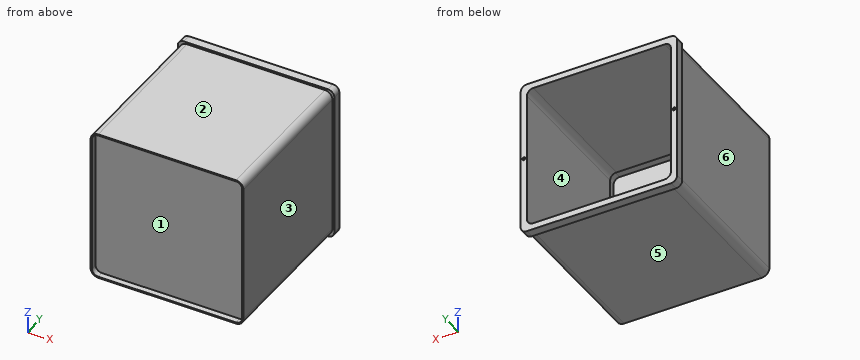
from build123d import *

# Parameters (mm, degrees)
EXTRUDE_1_DEPTH   = 125
EXTRUDE_1_2_DEPTH = 1
EXTRUDE_2_DEPTH   = 115
SKETCH_5_R        = 1.25
EXTRUDE_3_DEPTH   = 1
EXTRUDE_4_REACH   = 155.093
EXTRUDE_START     = -1
EXTRUDE_5_DEPTH   = 1


with BuildPart() as part:
    # Sketch 1 → Extrude 1 (new body)
    with BuildSketch(Plane(origin=(0, 0, 0), x_dir=(1, 0, 0), z_dir=(0, 1, 0))):
        with BuildLine():
            Line((55, -61), (-55, -61))
            ThreePointArc((-55, -61), (-59.242640687, -59.242640687), (-61, -55))
            Line((-61, -55), (-61, 55))
            ThreePointArc((-61, 55), (-59.242640687, 59.242640687), (-55, 61))
            Line((-55, 61), (55, 61))
            ThreePointArc((55, 61), (59.242640687, 59.242640687), (61, 55))
            Line((61, 55), (61, -55))
            ThreePointArc((61, -55), (59.242640687, -59.242640687), (55, -61))
        make_face()
        with BuildLine():
            Line((55, -60), (-55, -60))
            ThreePointArc((-55, -60), (-58.535533906, -58.535533906), (-60, -55))
            Line((-60, -55), (-60, 55))
            ThreePointArc((-60, 55), (-58.535533906, 58.535533906), (-55, 60))
            Line((-55, 60), (55, 60))
            ThreePointArc((55, 60), (58.535533906, 58.535533906), (60, 55))
            Line((60, 55), (60, -55))
            ThreePointArc((60, -55), (58.535533906, -58.535533906), (55, -60))
        make_face(mode=Mode.SUBTRACT)
    extrude(amount=EXTRUDE_1_DEPTH)

    # Sketch 2 → Extrude 1 2 (add)
    with BuildSketch(Plane(origin=(0, 5, 0), x_dir=(1, 0, 0), z_dir=(0, 1, 0))):
        with BuildLine():
            Line((-60, 55), (-60, -55))
            ThreePointArc((-60, -55), (-58.535533906, -58.535533906), (-55, -60))
            Line((-55, -60), (55, -60))
            ThreePointArc((55, -60), (58.535533906, -58.535533906), (60, -55))
            Line((60, -55), (60, 55))
            ThreePointArc((60, 55), (58.535533906, 58.535533906), (55, 60))
            Line((55, 60), (-55, 60))
            ThreePointArc((-55, 60), (-58.535533906, 58.535533906), (-60, 55))
        make_face()
    extrude(amount=EXTRUDE_1_2_DEPTH)



with BuildPart() as body_2:
    # Sketch 4 → Extrude 2 (new body)
    with BuildSketch(Plane(origin=(0, 15, 0), x_dir=(1, 0, 0), z_dir=(0, 1, 0))):
        with BuildLine():
            Line((-52.5, 58.5), (52.5, 58.5))
            ThreePointArc((52.5, 58.5), (56.742640687, 56.742640687), (58.5, 52.5))
            Line((58.5, 52.5), (58.5, -52.5))
            ThreePointArc((58.5, -52.5), (56.742640687, -56.742640687), (52.5, -58.5))
            Line((52.5, -58.5), (-52.5, -58.5))
            ThreePointArc((-52.5, -58.5), (-56.742640687, -56.742640687), (-58.5, -52.5))
            Line((-58.5, -52.5), (-58.5, 52.5))
            ThreePointArc((-58.5, 52.5), (-56.742640687, 56.742640687), (-52.5, 58.5))
        make_face()
        with BuildLine():
            Line((-52.5, 57.5), (52.5, 57.5))
            ThreePointArc((52.5, 57.5), (56.035533906, 56.035533906), (57.5, 52.5))
            Line((57.5, 52.5), (57.5, -52.5))
            ThreePointArc((57.5, -52.5), (56.035533906, -56.035533906), (52.5, -57.5))
            Line((52.5, -57.5), (-52.5, -57.5))
            ThreePointArc((-52.5, -57.5), (-56.035533906, -56.035533906), (-57.5, -52.5))
            Line((-57.5, -52.5), (-57.5, 52.5))
            ThreePointArc((-57.5, 52.5), (-56.035533906, 56.035533906), (-52.5, 57.5))
        make_face(mode=Mode.SUBTRACT)
    extrude(amount=EXTRUDE_2_DEPTH)

    # Sketch 5 → Extrude 3 (add)
    with BuildSketch(Plane(origin=(0, 130, 0), x_dir=(1, 0, 0), z_dir=(0, 1, 0))):
        with BuildLine():
            Line((-57.5, 62.5), (57.5, 62.5))
            ThreePointArc((57.5, 62.5), (61.035533906, 61.035533906), (62.5, 57.5))
            Line((62.5, 57.5), (62.5, -57.5))
            ThreePointArc((62.5, -57.5), (61.035533906, -61.035533906), (57.5, -62.5))
            Line((57.5, -62.5), (-57.5, -62.5))
            ThreePointArc((-57.5, -62.5), (-61.035533906, -61.035533906), (-62.5, -57.5))
            Line((-62.5, -57.5), (-62.5, 57.5))
            ThreePointArc((-62.5, 57.5), (-61.035533906, 61.035533906), (-57.5, 62.5))
        make_face()
        with Locations(Location((-60, 0, 0), (0, 0, 270))):
            Circle(SKETCH_5_R, mode=Mode.SUBTRACT)
        with Locations(Location((60, 0, 0), (0, 0, 270))):
            Circle(SKETCH_5_R, mode=Mode.SUBTRACT)
        with BuildLine():
            Line((-57.5, 52.5), (-57.5, -52.5))
            ThreePointArc((-57.5, -52.5), (-56.035533906, -56.035533906), (-52.5, -57.5))
            Line((-52.5, -57.5), (52.5, -57.5))
            ThreePointArc((52.5, -57.5), (56.035533906, -56.035533906), (57.5, -52.5))
            Line((57.5, -52.5), (57.5, 52.5))
            ThreePointArc((57.5, 52.5), (56.035533906, 56.035533906), (52.5, 57.5))
            Line((52.5, 57.5), (-52.5, 57.5))
            ThreePointArc((-52.5, 57.5), (-56.035533906, 56.035533906), (-57.5, 52.5))
        make_face(mode=Mode.SUBTRACT)
    extrude(amount=EXTRUDE_3_DEPTH)

    # Sketch 7 → Extrude 4 (add, up to next)
    with BuildSketch(Plane(origin=(0, 125, 0), x_dir=(1, 0, 0), z_dir=(0, 1, 0)), mode=Mode.PRIVATE) as extrude_4_sk1:
        with BuildLine():
            Line((62.5, -57.5), (62.5, 57.5))
            ThreePointArc((62.5, 57.5), (61.035533906, 61.035533906), (57.5, 62.5))
            Line((57.5, 62.5), (-57.5, 62.5))
            ThreePointArc((-57.5, 62.5), (-61.035533906, 61.035533906), (-62.5, 57.5))
            Line((-62.5, 57.5), (-62.5, -57.5))
            ThreePointArc((-62.5, -57.5), (-61.035533906, -61.035533906), (-57.5, -62.5))
            Line((-57.5, -62.5), (57.5, -62.5))
            ThreePointArc((57.5, -62.5), (61.035533906, -61.035533906), (62.5, -57.5))
        make_face()
        with BuildLine():
            Line((-56.5, -61.5), (56.5, -61.5))
            ThreePointArc((56.5, -61.5), (60.035533906, -60.035533906), (61.5, -56.5))
            Line((61.5, -56.5), (61.5, 56.5))
            ThreePointArc((61.5, 56.5), (60.035533906, 60.035533906), (56.5, 61.5))
            Line((56.5, 61.5), (-56.5, 61.5))
            ThreePointArc((-56.5, 61.5), (-60.035533906, 60.035533906), (-61.5, 56.5))
            Line((-61.5, 56.5), (-61.5, -56.5))
            ThreePointArc((-61.5, -56.5), (-60.035533906, -60.035533906), (-56.5, -61.5))
        make_face(mode=Mode.SUBTRACT)
    extrude_4_tool1 = extrude(extrude_4_sk1.sketch, amount=EXTRUDE_4_REACH, mode=Mode.PRIVATE) - body_2.part
    add(extrude_4_tool1.solids().sort_by_distance((60.910534, 125, 60.910534))[0])


with BuildPart() as part_1:
    add(part.part)

    add(body_2.part)  # Extrude 5 merges body 2
    # Sketch 8 → Extrude 5 (add)
    with BuildSketch(Plane(origin=(0, 125, 0), x_dir=(1, 0, 0), z_dir=(0, 1, 0)).offset(EXTRUDE_START)):
        with BuildLine():
            Line((-62.5, 57.5), (-62.5, -57.5))
            ThreePointArc((-62.5, -57.5), (-61.035533906, -61.035533906), (-57.5, -62.5))
            Line((-57.5, -62.5), (57.5, -62.5))
            ThreePointArc((57.5, -62.5), (61.035533906, -61.035533906), (62.5, -57.5))
            Line((62.5, -57.5), (62.5, 57.5))
            ThreePointArc((62.5, 57.5), (61.035533906, 61.035533906), (57.5, 62.5))
            Line((57.5, 62.5), (-57.5, 62.5))
            ThreePointArc((-57.5, 62.5), (-61.035533906, 61.035533906), (-62.5, 57.5))
        make_face()
        with BuildLine():
            Line((55, 61), (-55, 61))
            ThreePointArc((-55, 61), (-59.242640687, 59.242640687), (-61, 55))
            Line((-61, 55), (-61, -55))
            ThreePointArc((-61, -55), (-59.242640687, -59.242640687), (-55, -61))
            Line((-55, -61), (55, -61))
            ThreePointArc((55, -61), (59.242640687, -59.242640687), (61, -55))
            Line((61, -55), (61, 55))
            ThreePointArc((61, 55), (59.242640687, 59.242640687), (55, 61))
        make_face(mode=Mode.SUBTRACT)
    extrude(amount=EXTRUDE_5_DEPTH)


solid = part_1.part
Work out the finished part from the listing and answer in its coordinate system (mm). Face numbers are marked on the shaded views. A direction names the side the tool comes from. Give positions to 0.01 mm unless a question says otherwise; leave off trailing zeros. Write each loop counter-clockwise with the first axis right and the second up, starting at its lowest first coordinate (ties: lowest second). Pieces come first, ordered by that corner, then holes.
Q1. The part is cut by section C-C on x = -44.5. Give the vertices of the cut face in (y, z).
Answer:
outline: (0, -61) - (124, -61) - (124, -62.5) - (131, -62.5) - (131, -57.5) - (15, -57.5) - (15, -58.5) - (130, -58.5) - (130, -61.5) - (125, -61.5) - (125, -60) - (6, -60) - (6, 60) - (125, 60) - (125, 61.5) - (130, 61.5) - (130, 58.5) - (15, 58.5) - (15, 57.5) - (131, 57.5) - (131, 62.5) - (124, 62.5) - (124, 61) - (0, 61) - (0, 60) - (5, 60) - (5, -60) - (0, -60) - close
Q2. The part is cut by section B-B on y = 11. Give the vertices of the cut face in (x, z), and give its area (3 significant figures).
Answer:
outline: (-61, -55) arc R6 ccw to (-55, -61) - (55, -61) arc R6 ccw to (61, -55) - (61, 55) arc R6 ccw to (55, 61) - (-55, 61) arc R6 ccw to (-61, 55) - close; hole (-60, -55) arc R5 ccw to (-55, -60) - (55, -60) arc R5 ccw to (60, -55) - (60, 55) arc R5 ccw to (55, 60) - (-55, 60) arc R5 ccw to (-60, 55) - close
area: 475 mm2
Q3. A tool of negligible diameter and unlimited length cuts with its end or side. For the marked faces 4, 5 and 6, from which of +Z, -Z, +X, -X, +Y, -Y can it reach the whole face along a straight path? Write none if from no direction.
Answer:
face 4: +Y
face 5: -Z, +X, -X, -Y
face 6: +Z, -Z, -X, -Y
Q4. The part is cut by section A-A on y = 37.5. State how many separate pieces and enclosed holes the cut face has, and give its area (3 significant figures).
Answer:
separate pieces: 2
enclosed holes: 2
area: 929 mm2
Q5. For a pull along Z with two mould halves and no side action, classify the marked faces 1, 2 and 3 as released by +Z, released by -Z, zero draft, split by the parting line, or undercut.
Answer:
face 1: undercut
face 2: released by +Z
face 3: zero draft
Q6. Given pin 1 (6 mm diameter, centred on y = 16, z = -25.5, fed in from +X); pin 2 (12 mm diameter, centred on x = -18.5, z = 30.5, fed in from +Y); pin 3 (1.5 mm diameter, centred on x = 23, z = 4.5, fed in from -Y), each flat-ended and moving along its own axis, determine where each tip first touches the part or whether it passes through.
Answer:
pin 1: stops at x = 61
pin 2: stops at y = 6
pin 3: stops at y = 5
Q7. Straight lines are drawn through the part: L1, parallel to X at y = 63.5, z = 35; L2, parallel to X at y = 130.2, z = 0. For each, find the intervals that lie inside material, in ascending order.
Answer:
L1: x = -61 to -60, -58.5 to -57.5, 57.5 to 58.5, 60 to 61
L2: x = -62.5 to -61.25, -58.75 to -57.5, 57.5 to 58.75, 61.25 to 62.5
